Build history of the part. All positions in model axes, mm. Face numbers are marked on the shaded views. Coordinates: 2 decimals unless noted, no trailing zeros. Loops run counter-clockwise (first coordinate to the right, second up) from the corner with the lowest first, then second, coordinate; pieces in that order, holes last. Notation, with made-up numbers: (79.25, 61.5) -> (126.25, 61.5) arc R15 cw to (126.25, 79.5) -> close; hole circle Ø1 at (68.5, 26.25). An arc over 180 degrees is marked (long way). One line per item, written item: value. Start each with the question number.
```python
from build123d import *

# Parameters (mm, degrees)
SKETCH1_W                                   = 48
SKETCH1_H                                   = 43
BOSS_EXTRUDE1_DEPTH                         = 5
FILLET1_R                                   = 4
CSK_FOR_1_4_FLAT_HEAD_MACHINE_SCREW_2_COUNT = 2
CSK_FOR_1_4_FLAT_HEAD_MACHINE_SCREW_2_PITCH = 29
CUT_EXTRUDE2_DEPTH                          = 55


with BuildPart() as part:
    # Sketch1 → Boss-Extrude1 (new body)
    with BuildSketch(Plane(origin=(0, 0, 0), x_dir=(1, 0, 0), z_dir=(0, 1, 0))):
        Rectangle(SKETCH1_W, SKETCH1_H)
    extrude(amount=BOSS_EXTRUDE1_DEPTH)

    # Fillet1
    fillet1_edges = [part.edges().sort_by_distance(p)[0] for p in [
        (24, 2.5, 21.5),
        (-24, 2.5, 21.5),
        (-24, 2.5, -21.5),
        (24, 2.5, -21.5),
    ]]
    fillet(fillet1_edges, radius=FILLET1_R)

    # Sketch3 → CSK for 1/4 Flat Head Machine Screw (100)1 (revolve, cut)
    with BuildSketch(Plane(origin=(17, 5, 14.5), x_dir=(0, 0, 1), z_dir=(1, 0, 0))):
        Polygon((0, 0), (0, 30), (2.032, 28.779051222), (2.032, 2.237878716), (4.699, 0), align=None)
    csk_for_1_4_flat_head_machine_screw_100 = revolve(axis=Axis((17, 11.35, 14.5), (0, -1, 0)), mode=Mode.SUBTRACT)

    # CSK for 1_4 Flat Head Machine Screw  2: CSK for 1/4 Flat Head Machine Screw (100)1 ×2
    with Locations(*[(0, 0, -i * CSK_FOR_1_4_FLAT_HEAD_MACHINE_SCREW_2_PITCH) for i in range(1, CSK_FOR_1_4_FLAT_HEAD_MACHINE_SCREW_2_COUNT)]):
        add(csk_for_1_4_flat_head_machine_screw_100, mode=Mode.SUBTRACT)

    # Mirror1: CSK for 1/4 Flat Head Machine Screw (100)1 across plane
    add(csk_for_1_4_flat_head_machine_screw_100.mirror(Plane(origin=(0, 0, 0), x_dir=(0, 0, 1), z_dir=(1, 0, 0))), mode=Mode.SUBTRACT)

    # Mirror1 copy 1 sketch → Mirror1 copy 1 (revolve, cut)
    with BuildSketch(Plane(origin=(-17, 5, -14.5), x_dir=(0, 0, 1), z_dir=(-1, 0, 0))):
        Polygon((0, 0), (0, -30), (2.032, -28.779051222), (2.032, -2.237878716), (4.699, 0), align=None)
    revolve(axis=Axis((-17, 11.35, -14.5), (0, 1, 0)), mode=Mode.SUBTRACT)

    # Sketch6 → Cut-Extrude2 (cut)
    with BuildSketch(Plane(origin=(24, 0, 0), x_dir=(0, 0, -1), z_dir=(1, 0, 0))):
        with BuildLine():
            Line((-5.196152423, 0), (5.196152423, 0))
            ThreePointArc((5.196152423, 0), (0, 3), (-5.196152423, 0))
        make_face()
    extrude(amount=-CUT_EXTRUDE2_DEPTH, mode=Mode.SUBTRACT)


solid = part.part
```
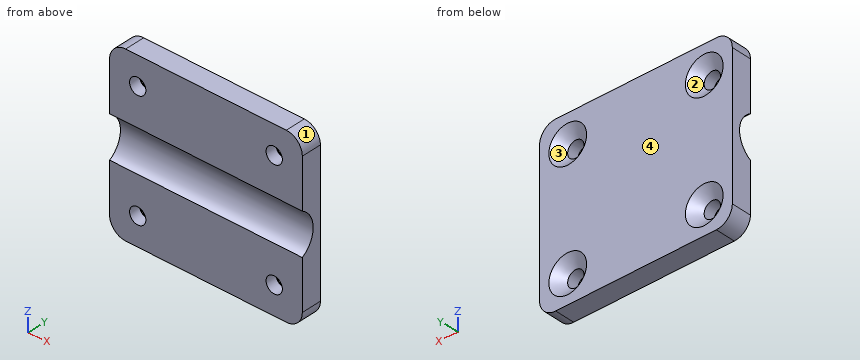
Item 1: Drop flat-ended pins along their axis: pin 1 Ø4.5 at (x, z) = (-17, -14.5) entering from -Y; pin 2 Ø6.5 at (x, z) = (-17, 14.5) entering from +Y; pin 3 Ø3 at (x, z) = (-7, 3.5) entering from -Y. Give the stop position or say it passes through.
Item 2: Probe probe 1 along X at (y, z) = (2.1, 14.5); probe 2 along Z at (x, y) = (17, 1); probe 3 along Z at (x, y) = (17, 0.6). List the from-to ranges inside material, lowest first.
Item 3: Two-plate mould, pull along X, no slides. Class the marked faces 1, 2, 3 and 4: +X half, -X half, draft (parallel to the pull), parting line (faces both ways), or undercut.
Item 4: Band-saw the part on D-D, the plane y = 4.45. List the corners of the cut face in (x, z).
Item 5: Band-saw the part on A-A, the plane z = -14.5. List the corners of the cut face in (x, y), and give its area (3 significant figures).
Item 6: Band-saw the part on C-C, the plane x = -17. List the corners of the cut face in (y, z).
Item 7: Band-saw the part on B-B, the plane y = 1.55. List the corners of the cut face in (x, z), and give its area (3 significant figures).
Worked out:
1. pin 1: stops at y = 0
1. pin 2: stops at y = 3.78
1. pin 3: stops at y = 0.32
2. probe 1: x = -24 to -19.03, -14.97 to 14.97, 19.03 to 24
2. probe 2: z = -21.5 to -16.53, -12.47 to -4.47, 4.47 to 12.47, 16.53 to 21.5
2. probe 3: z = -21.5 to -16.53, -12.47 to -4.8, 4.8 to 12.47, 16.53 to 21.5
3. face 1: +X half
3. face 2: undercut
3. face 3: undercut
3. face 4: draft
4. outline: (-24, -17.5) arc R4 ccw to (-20, -21.5) -> (20, -21.5) arc R4 ccw to (24, -17.5) -> (24, 17.5) arc R4 ccw to (20, 21.5) -> (-20, 21.5) arc R4 ccw to (-24, 17.5) -> close; hole circle Ø8.09 at (-17, -14.5); hole circle Ø8.09 at (-17, 14.5); hole circle Ø8.09 at (17, -14.5); hole circle Ø8.09 at (17, 14.5)
5. outline: (-24, 0) -> (-19.03, 0) -> (-19.03, 2.76) -> (-21.7, 5) -> (-24, 5) -> close; (-14.97, 0) -> (14.97, 0) -> (14.97, 2.76) -> (12.3, 5) -> (-12.3, 5) -> (-14.97, 2.76) -> close; (19.03, 0) -> (24, 0) -> (24, 5) -> (21.7, 5) -> (19.03, 2.76) -> close
5. area: 187 mm²
6. outline: (0, -21.5) -> (5, -21.5) -> (5, -19.2) -> (2.76, -16.53) -> (0, -16.53) -> close; (0, -12.47) -> (2.76, -12.47) -> (5, -9.8) -> (5, 9.8) -> (2.76, 12.47) -> (0, 12.47) -> (0, 5.2) arc R6 cw to (0, -5.2) -> close; (0, 16.53) -> (2.76, 16.53) -> (5, 19.2) -> (5, 21.5) -> (0, 21.5) -> close
7. outline: (-24, -17.5) arc R4 ccw to (-20, -21.5) -> (20, -21.5) arc R4 ccw to (24, -17.5) -> (24, -3.91) -> (-24, -3.91) -> close; (-24, 3.91) -> (24, 3.91) -> (24, 17.5) arc R4 ccw to (20, 21.5) -> (-20, 21.5) arc R4 ccw to (-24, 17.5) -> close; hole circle Ø4.06 at (-17, -14.5); hole circle Ø4.06 at (-17, 14.5); hole circle Ø4.06 at (17, -14.5); hole circle Ø4.06 at (17, 14.5)
7. area: 1,620 mm²
